Build history of the part. All positions in model axes, mm. A direction names the side the tool comes from. Give positions to 0.01 mm unless a question says otherwise; leave off trailing zeros. Write each loop counter-clockwise with the first axis right and the second up, starting at its lowest first coordinate (ties: lowest second). Pieces come first, ordered by that corner, then holes. Notation, with made-up numbers: M -22.5,-31 L -1.5,-31 A28 ccw -1.5,-11 Z; hole C 48,-25 d4. An arc over 180 degrees is marked long. Return JSON: item names as keys, results as strings. Group by question number.
Q1. Band-saw the part on B-B, the plane z = 17. Give the cut face in (x, y).
Q2. Band-saw the part on D-D, the plane y = 18. Give the cut face in (x, z).
Q3. Band-saw the part on A-A, the plane y = 4.5. Give the cut face in (x, z).
Q4. Wall check: probe 1 along Z at (x, y) = (17.5, 3); probe 2 along Z at (x, y) = (-17.5, 4); probe 3 along X at (y, z) = (11.25, -18). Give the ranges that are in metal, low to high.
Q5. Band-saw the part on C-C, the plane x = 17.5. Give the cut face in (y, z), then the cut area to 3 significant figures.
Q6. Pull direction Z, two halves, no side cores. Call faces 1 (the flat face through (16, 13, -16)), 2 (the flat face through (13.644, 6.409, 17.887)), 3 (the flat face through (-10, 10, -20)), 4 (the flat face through (0, 14.3, 2)): +Z half, -Z half, draft (parallel to the pull), parting line (faces both ways), or undercut.
Q7. Tool access for faces 5 (the flat face through (17.887, 6.409, -13.644)), 6 (the flat face through (-16, 13, 16)), 7 (the cylindrical face through (2.93, 16.84, -11.68)), 8 (the flat face through (13.6, 6.41, -17.84)), 9 (the flat face through (-18.21, 6.41, 13.97)): list every direction of +Z, -Z, +X, -X, +Y, -Y with a clear straight run to the whole face (end or side of a thin tool).
Q8. Flat gauge pins, fed straight in: pin 1 Ø8 at (x, z) = (-2, -1) entering from +Y; pin 2 Ø5 at (x, y) = (0, 3.5) entering from +Z; pin 3 Ø3 at (y, z) = (12.5, -10.5) entering from -X; pin 4 Ø2.5 at (x, z) = (-17.5, 17.5) entering from -Y. Where does each tip first touch, or does it go through?
from build123d import *

# Parameters (mm, degrees)
F0_R     = 1.7
F1_DEPTH = 13
F2_DEPTH = 19.3
F3_R     = 13.5
F4_DEPTH = 5


# Not quite as in the source:
# - ends of sketch curves that miss each other by under 0.0002 mm in the source are joined


with BuildPart() as f1:
    # F0 (on Front) → F1 (new body)
    with BuildSketch(Plane.XZ):
        with BuildLine():
            Line((-20.2, -20), (0, -20))
            ThreePointArc((0, -20), (6.2422337367, -19.0009083461), (11.8608111105, -16.1034517977))
            ThreePointArc((11.8608111105, -16.1034517977), (14.1421356237, -14.1421356237), (16.1034517977, -11.8608111105))
            ThreePointArc((16.1034517977, -11.8608111105), (20, 0), (16.1034517977, 11.8608111105))
            ThreePointArc((16.1034517977, 11.8608111105), (14.1421356237, 14.1421356237), (11.8608111105, 16.1034517977))
            ThreePointArc((11.8608111105, 16.1034517977), (0.0300507716, 19.9999774238), (-11.8123654956, 16.1390216989))
            Line((-11.8123654956, 16.1390216989), (-11.8608644463, 16.1035246693))
            Line((-11.8608644463, 16.1035246693), (-16.7602440212, 12.517603334))
            Line((-16.7602440212, 12.517603334), (-20.2, 10))
            Line((-20.2, 10), (-20.2, -20))
        make_face()
        with BuildLine():
            ThreePointArc((16.1034517977, -11.8608111105), (14.1421356237, -14.1421356237), (11.8608111105, -16.1034517977))
            Line((11.8608111105, -16.1034517977), (15.3786796564, -19.6213203436))
            ThreePointArc((15.3786796564, -19.6213203436), (19.6213203436, -19.6213203436), (19.6213203436, -15.3786796564))
            Line((19.6213203436, -15.3786796564), (16.1034517977, -11.8608111105))
        make_face()
        with Locations((17.5, -17.5)):
            Circle(F0_R, mode=Mode.SUBTRACT)
        with BuildLine():
            ThreePointArc((11.8608111105, 16.1034517977), (14.1421356237, 14.1421356237), (16.1034517977, 11.8608111105))
            Line((16.1034517977, 11.8608111105), (19.6213203436, 15.3786796564))
            ThreePointArc((19.6213203436, 15.3786796564), (19.6213203436, 19.6213203436), (15.3786796564, 19.6213203436))
            Line((15.3786796564, 19.6213203436), (11.8608111105, 16.1034517977))
        make_face()
        with Locations((17.5, 17.5)):
            Circle(F0_R, mode=Mode.SUBTRACT)
        with BuildLine():
            Line((-19.6213203436, 15.3786796564), (-16.7602440212, 12.517603334))
            Line((-16.7602440212, 12.517603334), (-11.8608644463, 16.1035246693))
            Line((-11.8608644463, 16.1035246693), (-15.3786796564, 19.6213203436))
            ThreePointArc((-15.3786796564, 19.6213203436), (-19.6213203436, 19.6213203436), (-19.6213203436, 15.3786796564))
        make_face()
        with Locations((-17.5, 17.5)):
            Circle(F0_R, mode=Mode.SUBTRACT)
    extrude(amount=-F1_DEPTH)

    # F0 (on Front) → F2 (join)
    with BuildSketch(Plane.XZ):
        with BuildLine():
            Line((-20.2, -20), (0, -20))
            ThreePointArc((0, -20), (6.2422337367, -19.0009083461), (11.8608111105, -16.1034517977))
            ThreePointArc((11.8608111105, -16.1034517977), (14.1421356237, -14.1421356237), (16.1034517977, -11.8608111105))
            ThreePointArc((16.1034517977, -11.8608111105), (20, 0), (16.1034517977, 11.8608111105))
            ThreePointArc((16.1034517977, 11.8608111105), (14.1421356237, 14.1421356237), (11.8608111105, 16.1034517977))
            ThreePointArc((11.8608111105, 16.1034517977), (0.0300507716, 19.9999774238), (-11.8123654956, 16.1390216989))
            Line((-11.8123654956, 16.1390216989), (-11.8608644463, 16.1035246693))
            Line((-11.8608644463, 16.1035246693), (-16.7602440212, 12.517603334))
            Line((-16.7602440212, 12.517603334), (-20.2, 10))
            Line((-20.2, 10), (-20.2, -20))
        make_face()
    extrude(amount=-F2_DEPTH)

    # F3 (on face) → F4 (cut)
    with BuildSketch(Plane(origin=(0, 19.3, 0), x_dir=(-1, 0, 0), z_dir=(0, 1, 0))):
        with Locations((0, 1.5)):
            Circle(F3_R)
    extrude(amount=-F4_DEPTH, mode=Mode.SUBTRACT)


solid = f1.part
From the geometry:
{
 "1": {"outline": "M -20.46,0 L -19.12,0 L -19.12,13 L -20.46,13 Z; M -15.88,0 L -12.76,0 L -12.76,13 L -15.88,13 Z; M -10.54,0 L 10.54,0 L 10.54,19.3 L -10.54,19.3 Z; M 12.76,0 L 15.88,0 L 15.88,13 L 12.76,13 Z; M 19.12,0 L 20.46,0 L 20.46,13 L 19.12,13 Z"},
 "2": {"outline": "M -20.2,-20 L 0,-20 A20 ccw long -11.81,16.14 L -20.2,10 Z; hole C 0,1.5 d27"},
 "3": {"outline": "M -20.2,-20 L 0,-20 A20 ccw 11.86,-16.1 L 15.38,-19.62 A3 ccw 19.62,-15.38 L 16.1,-11.86 A20 ccw 16.1,11.86 L 19.62,15.38 A3 ccw 15.38,19.62 L 11.86,16.1 A20 ccw -11.81,16.14 L -11.86,16.1 L -15.38,19.62 A3 ccw -19.62,15.38 L -16.76,12.52 L -20.2,10 Z; hole C -17.5,17.5 d3.4; hole C 17.5,-17.5 d3.4; hole C 17.5,17.5 d3.4"},
 "4": {"probe 1": "z = -20.5 to -19.2, -15.8 to -13.26, -9.68 to 9.68, 13.26 to 15.8, 19.2 to 20.5", "probe 2": "z = -20 to 11.98, 13.26 to 15.8, 19.2 to 20.5", "probe 3": "x = -20.2 to 8.72, 13.76 to 15.88, 19.12 to 20.46"},
 "5": {"outline": "M 0,-20.5 L 13,-20.5 L 13,-19.2 L 0,-19.2 Z; M 0,-15.8 L 13,-15.8 L 13,-13.26 L 0,-13.26 Z; M 0,-9.68 L 19.3,-9.68 L 19.3,9.68 L 0,9.68 Z; M 0,13.26 L 13,13.26 L 13,15.8 L 0,15.8 Z; M 0,19.2 L 13,19.2 L 13,20.5 L 0,20.5 Z", "area": "474 mm^2"},
 "6": {"face 1": "draft", "face 2": "+Z half", "face 3": "-Z half", "face 4": "undercut"},
 "7": {"face 5": "+X, +Y, -Y", "face 6": "+Z, -X, +Y", "face 7": "+Y", "face 8": "-Z, +Y, -Y", "face 9": "-X, +Y, -Y"},
 "8": {"pin 1": "stops at y = 14.3", "pin 2": "stops at z = 20", "pin 3": "stops at x = -20.2", "pin 4": "passes through"}
}
